Check sheet for the modelled part. Datum: model origin and axes. Units: mm. Coordinates: 2 decimals unless noted, no trailing zeros. Write each loop counter-clockwise with the first axis right and the second up, starting at its lowest first coordinate (ties: lowest second). Pieces come first, ordered by that corner, then holes. Notation, with made-up numbers: (62, -7.75) - (96, -7.75) arc R17 cw to (96, 17.25) - close; hole circle Ø6 at (88, 40). An arc over 180 degrees is marked (long way). Use one line per item in the form item = value. Start each with the question number.
1. Cross-section at B-B on x = -87. Record the boundary of the cut face in (y, z), then the cut area to 3 significant figures.
2. Cross-section at A-A on z = -11. Record the boundary of the cut face in (x, y), then the cut area to 3 significant figures.
3. Scan lines: line 1 along Z through (x, y) = (49, 2.5); line 2 along Z through (x, y) = (-32.5, 4.5); line 3 along X through (y, z) = (3.5, -17.5). Record each from-to range of solid material in increasing order.
4. Cross-section at C-C on x = 80. Record the boundary of the cut face in (y, z).
5. Go/stop test with flat-tipped pins: pin 1 Ø1 at (x, z) = (-9, 15) entering from +Y; pin 2 Ø0.9 at (x, z) = (3.5, -16.5) entering from +Y. Record where each tip stops, or that it passes through.
```python
from build123d import *

# Parameters (mm, degrees)
SKETCH_1_W               = 238
SKETCH_1_H               = 41
SKETCH_1_W_2             = 230
SKETCH_1_H_2             = 27
EXTRUDE_1_DEPTH          = 5
SKETCH_2_W               = 20
SKETCH_2_H               = 3
CUT_EXTRUDE_1_DEPTH      = 3
MIRROR_2_COPY_1_SKETCH_W = 20
MIRROR_2_COPY_1_SKETCH_H = 3
MIRROR_2_COPY_1_DEPTH    = 3
SKETCH_3_W               = 2.5
SKETCH_3_H               = 2.5
EXTRUDE_2_DEPTH          = 2.5
SKETCH_3_3_W             = 2.5
SKETCH_3_3_H             = 2.5
CUT_EXTRUDE_2_DEPTH      = 2.5


with BuildPart() as part:
    # 草图1 → 凸台-拉伸1 (new body)
    with BuildSketch(Plane(origin=(0, 0, 0), x_dir=(1, 0, 0), z_dir=(0, 1, 0))):
        Rectangle(SKETCH_1_W, SKETCH_1_H)
        Rectangle(SKETCH_1_W_2, SKETCH_1_H_2, mode=Mode.SUBTRACT)
    extrude(amount=EXTRUDE_1_DEPTH)

    # 草图2 → 切除-拉伸1 (cut)
    with BuildSketch(Plane(origin=(0, 5, 0), x_dir=(1, 0, 0), z_dir=(0, 1, 0))):
        with Locations((0, 17)):
            Rectangle(SKETCH_2_W, SKETCH_2_H)
        with Locations((46, 17)):
            Rectangle(SKETCH_2_W, SKETCH_2_H)
        with Locations((92, 17)):
            Rectangle(SKETCH_2_W, SKETCH_2_H)
    cut_extrude_1 = extrude(amount=-CUT_EXTRUDE_1_DEPTH, mode=Mode.SUBTRACT)

    # 镜向1: 切除-拉伸1 across plane
    add(cut_extrude_1.mirror(Plane.XY), mode=Mode.SUBTRACT)

    # 镜向2: 切除-拉伸1 across plane
    add(cut_extrude_1.mirror(Plane(origin=(0, 0, 0), x_dir=(0, 0, 1), z_dir=(1, 0, 0))), mode=Mode.SUBTRACT)

    # 镜向2 copy 1 sketch → 镜向2 copy 1 (cut)
    with BuildSketch(Plane(origin=(0, 5, 0), x_dir=(-1, 0, 0), z_dir=(0, 1, 0))):
        with Locations((0, 17)):
            Rectangle(MIRROR_2_COPY_1_SKETCH_W, MIRROR_2_COPY_1_SKETCH_H)
        with Locations((46, 17)):
            Rectangle(MIRROR_2_COPY_1_SKETCH_W, MIRROR_2_COPY_1_SKETCH_H)
        with Locations((92, 17)):
            Rectangle(MIRROR_2_COPY_1_SKETCH_W, MIRROR_2_COPY_1_SKETCH_H)
    extrude(amount=-MIRROR_2_COPY_1_DEPTH, mode=Mode.SUBTRACT)

    # 草图3 → 凸台-拉伸2 (add)
    with BuildSketch(Plane(origin=(0, 5, 0), x_dir=(1, 0, 0), z_dir=(0, 1, 0))):
        with Locations((-111.25, -19.25)):
            Rectangle(SKETCH_3_W, SKETCH_3_H)
        with Locations((111.25, 19.25)):
            Rectangle(SKETCH_3_W, SKETCH_3_H)
    extrude(amount=EXTRUDE_2_DEPTH)

    # 草图3<3> → 切除-拉伸2 (cut)
    with BuildSketch(Plane(origin=(0, 5, 0), x_dir=(1, 0, 0), z_dir=(0, 1, 0))):
        with Locations((-111.25, 19.25)):
            Rectangle(SKETCH_3_3_W, SKETCH_3_3_H)
        with Locations((111.25, -19.25)):
            Rectangle(SKETCH_3_3_W, SKETCH_3_3_H)
    extrude(amount=-CUT_EXTRUDE_2_DEPTH, mode=Mode.SUBTRACT)


solid = part.part
```
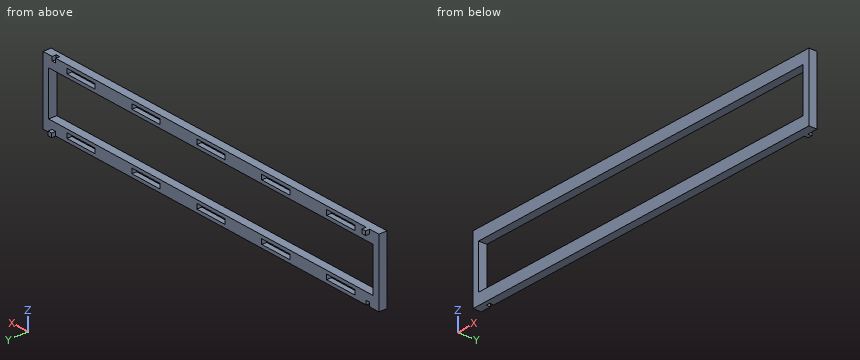
Final values:
q1.outline = (0, -20.5) - (5, -20.5) - (5, -18.5) - (2, -18.5) - (2, -15.5) - (5, -15.5) - (5, -13.5) - (0, -13.5) - close; (0, 13.5) - (5, 13.5) - (5, 15.5) - (2, 15.5) - (2, 18.5) - (5, 18.5) - (5, 20.5) - (0, 20.5) - close
q1.area = 52.0 mm²
q2.outline = (-119, 0) - (-115, 0) - (-115, 5) - (-119, 5) - close; (115, 0) - (119, 0) - (119, 5) - (115, 5) - close
q2.area = 40.0 mm²
q3.line_1 = -20.5 to -18.5, -15.5 to -13.5, 13.5 to 15.5, 18.5 to 20.5
q3.line_2 = -20.5 to -13.5, 13.5 to 20.5
q3.line_3 = -119 to -102, -82 to -56, -36 to -10, 10 to 36, 56 to 82, 102 to 119
q4.outline = (0, -20.5) - (5, -20.5) - (5, -13.5) - (0, -13.5) - close; (0, 13.5) - (5, 13.5) - (5, 20.5) - (0, 20.5) - close
q5.pin_1 = 5
q5.pin_2 = 2
